The drawing under review shows one solid part. Ordinate dimensions are in mm from its lowest x, y, z. A direction names the side the tool comes from. Coordinates: 2 decimals unless noted, no trailing zeros. Loops run counter-clockwise (first coordinate to the right, second up) from the corner with the lowest first, then second, coordinate; pieces in that order, holes last. Notation, with made-up numbers: M 30.25,89 L 61.25,89 A19 ccw 61.25,105 Z; hole C 12.5,88.25 d9. An arc over 180 degrees is marked long. Put each result on its own line as item: value.
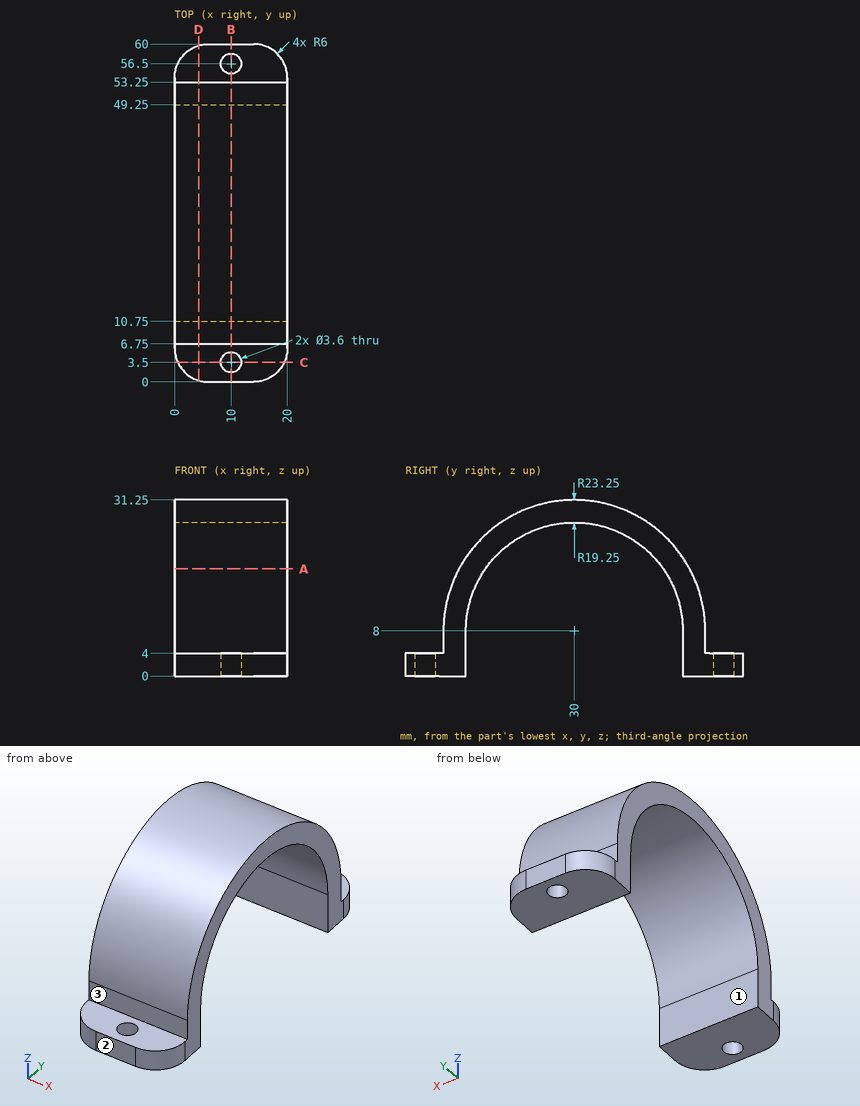
(1) Tool access review of the marked faces 1, 2 and 3: name each direction out of +Z, -Z, +X, -X, +Y, -Y from which nothing blocks a thin tool from reaching the whole face with its end or side.
Determined:
face 1: -Z, +X, -X
face 2: +Z, -Z, +X, -X, -Y
face 3: +Z, +X, -X, -Y
(2) Add section D-D (x = 4.25). Write out the cut boundary in (y, z), plus the area to 3 significant figures.
Determined:
outline: M 0.26,0 L 10.75,0 L 10.75,8 A19.25 cw 49.25,8 L 49.25,0 L 59.74,0 L 59.74,4 L 53.25,4 L 53.25,8 A23.25 ccw 6.75,8 L 6.75,4 L 0.26,4 Z
area: 383 mm^2
(3) Add section C-C (y = 3.5). Write out the cut boundary in (x, z).
Determined:
outline: M 0.55,0 L 8.2,0 L 8.2,4 L 0.55,4 Z; M 11.8,0 L 19.45,0 L 19.45,4 L 11.8,4 Z
(4) Add section B-B (x = 10). Write out the cut boundary in (y, z), plus the area to 3 significant figures.
Determined:
outline: M 0,0 L 1.7,0 L 1.7,4 L 0,4 Z; M 5.3,0 L 10.75,0 L 10.75,8 A19.25 cw 49.25,8 L 49.25,0 L 54.7,0 L 54.7,4 L 53.25,4 L 53.25,8 A23.25 ccw 6.75,8 L 6.75,4 L 5.3,4 Z; M 58.3,0 L 60,0 L 60,4 L 58.3,4 Z
area: 356 mm^2
(5) Add section A-A (z = 19). Write out the cut boundary in (x, y).
Determined:
outline: M 0,9.52 L 20,9.52 L 20,14.2 L 0,14.2 Z; M 0,45.8 L 20,45.8 L 20,50.48 L 0,50.48 Z
(6) For pin 1 (3 mm diameter, centred on x = 10, y = 3.5, fed in from -Z); pin 2 (10 mm diameter, centred on x = 10, y = 22.5, fed in from -Z); pin 3 (2 mm diameter, centred on x = 15, z = 6.5, fed in from -Y); pin 4 (8 mm diameter, centred on x = 5.5, y = 34, fed in from -Z), all flat-tipped, find the tip position at first contact; note any pin that passes through.
Determined:
pin 1: passes through
pin 2: stops at z = 22.64
pin 3: stops at y = 6.75
pin 4: stops at z = 25.51
(7) Wall thickness on line 1 along Y through (x, z) = (10, 2.35); line 2 along Y through (x, z) = (2.75, 8); line 3 along Z through (x, y) = (3.5, 3): over which ranges is each line inside the solid? List them lowest first. Write a range as [from, to].
Determined:
line 1: y = [0, 1.7], [5.3, 10.75], [49.25, 54.7], [58.3, 60]
line 2: y = [6.75, 10.75], [49.25, 53.25]
line 3: z = [0, 4]
